Part model, mm, in its own coordinate system. A direction names the side the tool comes from. Round coordinates to 2 decimals unless told otherwise and drop trailing zeros. Loops run counter-clockwise (first coordinate to the right, second up) from the corner with the lowest first, then second, coordinate; pieces in that order, holes last. Notation, with made-up numbers: (-39.5, 17) - (-3.5, 17) arc R20 cw to (-3.5, 37) - close; hole circle Ø1 at (-5.5, 32.5). An arc over 180 degrees is marked (long way). Put each result on its own line as item: value.
from build123d import *

# Parameters (mm, degrees)
SKETCH1_W           = 42
SKETCH1_H           = 24
BOSS_EXTRUDE1_DEPTH = 5
SKETCH2_W           = 33.4
SKETCH2_H           = 15.4
CUT_EXTRUDE1_DEPTH  = 6
SKETCH3_W           = 15
SKETCH3_H           = 32
BOSS_EXTRUDE2_DEPTH = 5
SKETCH4_W           = 25.4
SKETCH4_H           = 9.3
BOSS_EXTRUDE3_DEPTH = 5
SKETCH5_R           = 1.75
CUT_EXTRUDE2_DEPTH  = 6
SKETCH6_R           = 1.115
CUT_EXTRUDE3_DEPTH  = 6


with BuildPart() as part:
    # Sketch1 → Boss-Extrude1 (new body)
    with BuildSketch(Plane(origin=(0, 0, 0), x_dir=(1, 0, 0), z_dir=(0, 1, 0))):
        with Locations((21, 12)):
            Rectangle(SKETCH1_W, SKETCH1_H)
    extrude(amount=BOSS_EXTRUDE1_DEPTH)

    # Sketch2 → Cut-Extrude1 (cut, through all)
    with BuildSketch(Plane(origin=(0, 5, 0), x_dir=(1, 0, 0), z_dir=(0, 1, 0))):
        with Locations((21, 12)):
            Rectangle(SKETCH2_W, SKETCH2_H)
    extrude(amount=-CUT_EXTRUDE1_DEPTH, mode=Mode.SUBTRACT)

    # Sketch3 → Boss-Extrude2 (add)
    with BuildSketch(Plane(origin=(0, 5, 0), x_dir=(1, 0, 0), z_dir=(0, 1, 0))):
        with Locations((21, -16)):
            Rectangle(SKETCH3_W, SKETCH3_H)
    extrude(amount=-BOSS_EXTRUDE2_DEPTH)

    # Sketch4 → Boss-Extrude3 (add)
    with BuildSketch(Plane(origin=(0, 5, 0), x_dir=(1, 0, 0), z_dir=(0, 1, 0))):
        with Locations((21, -36.65)):
            Rectangle(SKETCH4_W, SKETCH4_H)
    extrude(amount=-BOSS_EXTRUDE3_DEPTH)

    # Sketch5 → Cut-Extrude2 (cut, through all)
    with BuildSketch(Plane(origin=(0, 5, 0), x_dir=(1, 0, 0), z_dir=(0, 1, 0))):
        with Locations((13.3, -36.81777032)):
            Circle(SKETCH5_R)
        with Locations((28.7, -36.81777032)):
            Circle(SKETCH5_R)
    extrude(amount=-CUT_EXTRUDE2_DEPTH, mode=Mode.SUBTRACT)

    # Sketch6 → Cut-Extrude3 (cut, through all)
    with BuildSketch(Plane(origin=(0, 5, 0), x_dir=(1, 0, 0), z_dir=(0, 1, 0))):
        with Locations((3, 12)):
            Circle(SKETCH6_R)
        with Locations((39, 12)):
            Circle(SKETCH6_R)
    extrude(amount=-CUT_EXTRUDE3_DEPTH, mode=Mode.SUBTRACT)


solid = part.part
1. Band-saw the part on B-B (x = 35.5). List the corners of the cut face in (y, z).
A:
outline: (0, -24) - (5, -24) - (5, -19.7) - (0, -19.7) - close; (0, -4.3) - (5, -4.3) - (5, 0) - (0, 0) - close
2. Band-saw the part on A-A (z = -12). List the corners of the cut face in (x, y) (3 decimals).
A:
outline: (0, 0) - (1.885, 0) - (1.885, 5) - (0, 5) - close; (4.115, 0) - (4.3, 0) - (4.3, 5) - (4.115, 5) - close; (37.7, 0) - (37.885, 0) - (37.885, 5) - (37.7, 5) - close; (40.115, 0) - (42, 0) - (42, 5) - (40.115, 5) - close
3. Pin check, flat tips, straight feed: P1, Ø3, axis at x = 28.7, z = 36.82, coming from the +Y side; P2, Ø1.5, axis at y = 2, z = 19, coming from the +X side; P3, Ø1.5, axis at y = 2, z = 32, coming from the +X side; P4, Ø1.5, axis at x = 35, y = 1.5, coming from the +Z side. Stop position of each tip, or through.
A:
P1: passes through
P2: stops at x = 28.5
P3: stops at x = 33.7
P4: stops at z = 0
4. Probe line 1 along X through (y, z) = (1.45, -12) (3 decimals); line 2 along Z through (x, y) = (31, 2.4); line 3 along Z through (x, y) = (13.3, 1.3). List the from-to ranges inside material, lowest first. Write a range as [from, to].
A:
line 1: x = [0, 1.885], [4.115, 4.3], [37.7, 37.885], [40.115, 42]
line 2: z = [-24, -19.7], [-4.3, 0], [32, 41.3]
line 3: z = [-24, -19.7], [-4.3, 0], [32, 35.07], [38.57, 41.3]
5. Band-saw the part on D-D (x = 12.5). List the corners of the cut face in (y, z), plus the area to 3 significant figures.
A:
outline: (0, -24) - (5, -24) - (5, -19.7) - (0, -19.7) - close; (0, -4.3) - (5, -4.3) - (5, 0) - (0, 0) - close; (0, 32) - (5, 32) - (5, 35.26) - (0, 35.26) - close; (0, 38.37) - (5, 38.37) - (5, 41.3) - (0, 41.3) - close
area: 73.9 mm²
6. Band-saw the part on C-C (y = 2). List the corners of the cut face in (x, z) (3 decimals).
A:
outline: (0, -24) - (42, -24) - (42, 0) - (28.5, 0) - (28.5, 32) - (33.7, 32) - (33.7, 41.3) - (8.3, 41.3) - (8.3, 32) - (13.5, 32) - (13.5, 0) - (0, 0) - close; hole circle Ø2.23 at (3, -12); hole (4.3, -19.7) - (37.7, -19.7) - (37.7, -4.3) - (4.3, -4.3) - close; hole circle Ø3.5 at (13.3, 36.818); hole circle Ø3.5 at (28.7, 36.818); hole circle Ø2.23 at (39, -12)
7. Two-plate mould, pull along Z, no slides. Class faces 5 (the flat face through (8.3, 3, 37)), 6 (the flat face through (21, 2, -24)), 7 (the flat face through (21, 3, -4.3)): pulls with the +Z half, pulls with the -Z half, needs draft (parallel to the pull), parting line crosses it, or undercut.
A:
face 5: needs draft
face 6: pulls with the -Z half
face 7: undercut
8. Tool access for faces 1 (the flat face through (33.7, 3, 37)), 2 (the flat face through (13.5, 3, 16)), 3 (the flat face through (4.3, 3, -12)), 4 (the flat face through (28.5, 3, 16)): list every direction of +Z, -Z, +X, -X, +Y, -Y with a clear straight run to the whole face (end or side of a thin tool).
A:
face 1: +Z, +X, +Y, -Y
face 2: -X, +Y, -Y
face 3: +Y, -Y
face 4: +X, +Y, -Y
